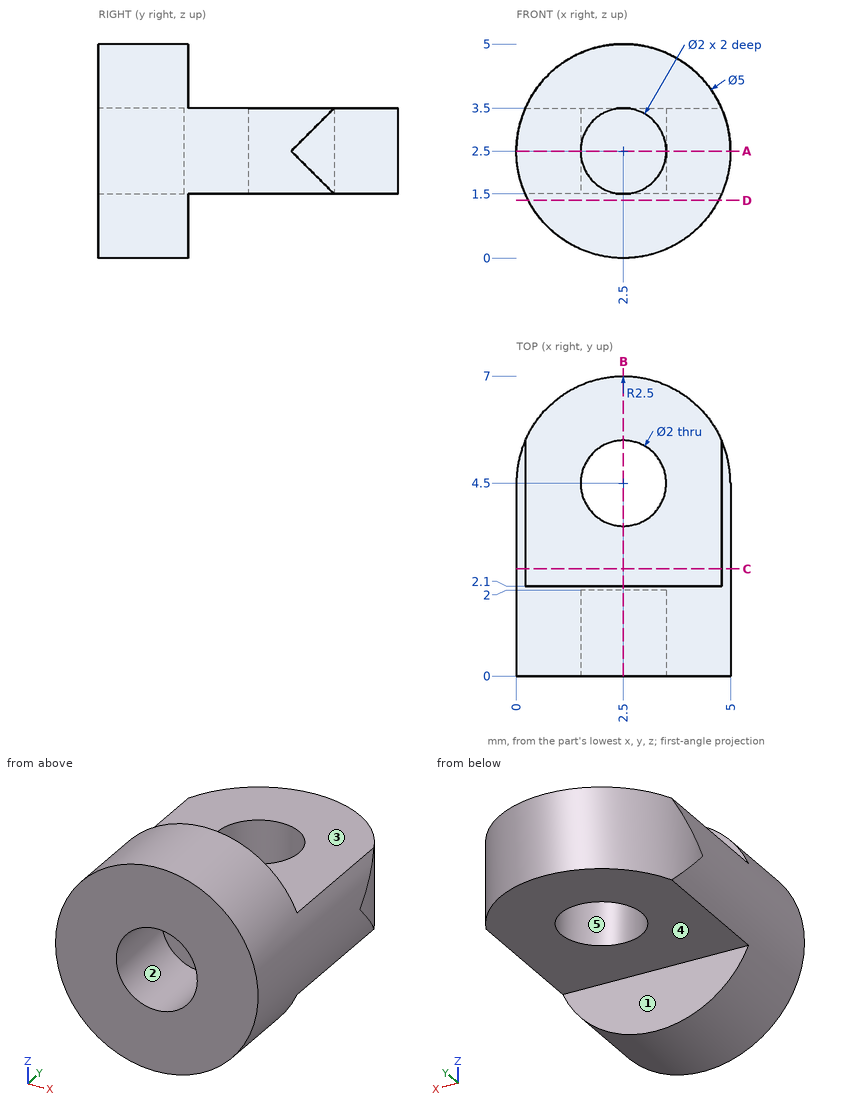
Part print with two shaded views. Sizes in mm from the minimum x, y, z corner. A direction names the side the tool comes from. Round coordinates to 2 decimals unless told otherwise and drop trailing zeros. Order: outer loops, then holes, each group sorted by start corner. A loop starts at its lowest first (then second) coordinate and runs counter-clockwise, first axis right, second up. Notation, with made-up numbers: (-10.75, -28) - (-2.75, -28) arc R31 cw to (-2.75, 9) - close; hole circle Ø4 at (-29.75, -26.75). An arc over 180 degrees is marked (long way). Answer in a Markdown table with one row per item. Add a question column.
(1) Band-saw the part on A-A on z = 2.5. List the corners of the cut face in (x, y), and give its area (3 significant figures).
(2) Band-saw the part on B-B on x = 2.5. List the corners of the cut face in (y, z), and give its area (3 significant figures).
(3) Mould opens along Z. For the marked faces 1, 2 and 3 say: +Z half, -Z half, draft (parallel to the pull), parting line (faces both ways), or undercut.
(4) 3-axis set-ups, long thin cutter, end or side, ignore diameter. For the marked faces 4 and 5: which of +Z, -Z, +X, -X, +Y, -Y reach the whole face in a straight line?
(5) Drop flat-ended pins along their axis: pin 1 Ø1.5 at (y, z) = (1.5, 4) entering from +X; pin 2 Ø3 at (x, y) = (2.5, 4.5) entering from -Z; pin 3 Ø1.2 at (x, z) = (1.5, 4.5) entering from +Y; pin 4 Ø1 at (x, z) = (3.5, 3) entering from -Y. Give the stop position or say it passes through.
(6) Band-saw the part on D-D on z = 1.35. List the corners of the cut face in (x, y).
(7) Band-saw the part on C-C on y = 2.5. List the corners of the cut face in (x, z).
(8) Probe L1, parallel to Y at x = 2.5, z = 2.5; L2, parallel to X at y = 0.7, z = 2.5; L3, parallel to Y at x = 3.25, z = 0.3. List the from-to ranges inside material, lowest first. Write a range as [from, to].
Data:
| question | item | result |
|---|---|---|
| 1 | outline | (0, 0) - (1.5, 0) - (1.5, 2) - (3.5, 2) - (3.5, 0) - (5, 0) - (5, 4.5) arc R2.5 ccw to (0, 4.5) - close; hole circle Ø2 at (2.5, 4.5) |
| 1 | area | 25.2 mm^2 |
| 2 | outline | (0, 0) - (2.1, 0) - (2.1, 1.5) - (3.5, 1.5) - (3.5, 3.5) - (2.1, 3.5) - (2.1, 5) - (0, 5) - (0, 3.5) - (2, 3.5) - (2, 1.5) - (0, 1.5) - close; (5.5, 1.5) - (7, 1.5) - (7, 3.5) - (5.5, 3.5) - close |
| 2 | area | 12.3 mm^2 |
| 3 | face 1 | draft |
| 3 | face 2 | undercut |
| 3 | face 3 | +Z half |
| 4 | face 4 | -Z, +X, -X, +Y |
| 4 | face 5 | +Z, -Z |
| 5 | pin 1 | stops at x = 4.88 |
| 5 | pin 2 | stops at z = 1.5 |
| 5 | pin 3 | stops at y = 2.1 |
| 5 | pin 4 | stops at y = 0 |
| 6 | outline | (0.28, 0) - (4.72, 0) - (4.72, 2.1) - (0.28, 2.1) - close |
| 7 | outline | (0.21, 1.5) - (4.79, 1.5) arc R2.5 ccw to (4.79, 3.5) - (0.21, 3.5) arc R2.5 ccw to start |
| 8 | L1 | y = [2, 3.5], [5.5, 7] |
| 8 | L2 | x = [0, 1.5], [3.5, 5] |
| 8 | L3 | y = [0, 2.1] |
